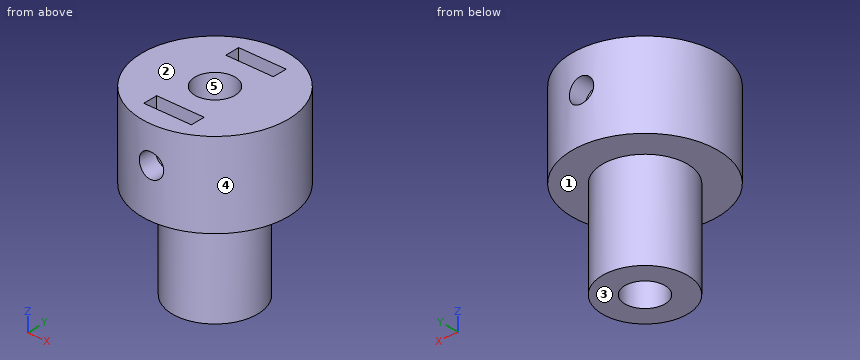
from build123d import *

# Parameters (mm, degrees)
SKETCH1_R           = 6
BOSS_EXTRUDE1_DEPTH = 15
SKETCH2_R           = 1.65
CUT_EXTRUDE1_DEPTH  = 18.23368794
SKETCH13_W          = 3.9
SKETCH13_H          = 1.2
CUT_EXTRUDE6_DEPTH  = 4.95
SKETCH4_R           = 1
CUT_EXTRUDE7_DEPTH  = 7.5
SKETCH19_R          = 6
SKETCH19_R_2        = 5.5
SKETCH19_R_3        = 3.5
CUT_EXTRUDE12_DEPTH = 8


with BuildPart() as part:
    # Sketch1 → Boss-Extrude1 (new body)
    with BuildSketch(Plane.XY):
        Circle(SKETCH1_R)
    extrude(amount=BOSS_EXTRUDE1_DEPTH)

    # Sketch2 → Cut-Extrude1 (cut, through all)
    with BuildSketch(Plane.XY.offset(15)):
        Circle(SKETCH2_R)
    extrude(amount=-CUT_EXTRUDE1_DEPTH, mode=Mode.SUBTRACT)

    # Sketch13 → Cut-Extrude6 (cut)
    with BuildSketch(Plane.XY.offset(15)):
        with Locations((0, 3.825)):
            Rectangle(SKETCH13_W, SKETCH13_H)
    cut_extrude6 = extrude(amount=-CUT_EXTRUDE6_DEPTH, mode=Mode.SUBTRACT)

    # Sketch4 → Cut-Extrude7 (cut, symmetric)
    with BuildSketch(Plane(origin=(0, 0, 0), x_dir=(1, 0, 0), z_dir=(0, 1, 0))):
        with Locations(Location((0, -12, 0), (0, 0, 270))):
            Circle(SKETCH4_R)
    extrude(amount=CUT_EXTRUDE7_DEPTH, both=True, mode=Mode.SUBTRACT)

    # Mirror1: Cut-Extrude6 across plane
    add(cut_extrude6.mirror(Plane.ZX), mode=Mode.SUBTRACT)

    # Sketch19 → Cut-Extrude12 (cut)
    # profile 1 of 2: a face of its own
    with BuildSketch(Plane(origin=(0, 0, 0), x_dir=(-1, 0, 0), z_dir=(0, 0, -1))):
        Circle(SKETCH19_R)
        Circle(SKETCH19_R_2, mode=Mode.SUBTRACT)
    # profile 2 of 2: a face of its own
    with BuildSketch(Plane(origin=(0, 0, 0), x_dir=(-1, 0, 0), z_dir=(0, 0, -1))):
        Circle(SKETCH19_R_2)
        Circle(SKETCH19_R_3, mode=Mode.SUBTRACT)
    extrude(amount=-CUT_EXTRUDE12_DEPTH, mode=Mode.SUBTRACT)


solid = part.part
Input: part model. Units: mm. Frame: model coordinates. Face numbers are marked on the shaded views. A direction names the side the tool comes from. Coordinates: 2 decimals unless noted, no trailing zeros. Write each loop counter-clockwise with the first axis right and the second up, starting at its lowest first coordinate (ties: lowest second). Pieces come first, ordered by that corner, then holes. Notation, with made-up numbers: M -22.75,10.5 L 26.25,10.5 A26 cw 26.25,37.5 Z; hole C 7,50 d9. An arc over 180 degrees is marked long. Answer as a JSON object with one key per item and string values. Group by question number.
(1) Ray query, line 1 along Y through (x, z) = (-1.5, 14.25) (3 decimals); line 2 along Y through (x, z) = (-0.5, 13.25) (3 decimals); line 3 along X through (y, z) = (-0.75, 9.5). Return the intervals inside material, ascending. Write a range as [from, to].
(2) Mould query, pull axis X, two halves, no side actions, for the marked faces 3, 4 and 5. Classes: pulls with the +X half, pulls with the -X half, needs draft (parallel to the pull), parting line crosses it, or undercut.
(3) Set-up query: the marked faces 1 and 2. Return all of +Z, -Z, +X, -X, +Y, -Y with unobstructed straight access to the full face (end or side cutting, diameter ignored); none if empty.
(4) Section A-A on y = 0. Output: boundary loops of the cut face in (x, z), plus the area to 3 significant figures.
(5) Section B-B on z = 12. Output: boundary loops of the cut face in (x, y) (3 decimals).
(6) Section C-C on x = 0. Give the number of separate pieces and of enclosed holes in the cut face, plus the area to 3 significant figures.
(7) Section D-D on z = 4.5. Output: boundary loops of the cut face in (x, y), plus the area to 3 significant figures.
(8) Contact query for flat-ended pins moving along their axis: P1, Ø1.2, axis at x = -0.5, z = 12, coming from the -Y side; P2, Ø2, axis at x = 2.5, z = 2.5, coming from the -Y side; P3, Ø0.6, axis at y = 3.5, z = 12.5, coming from the +X side. Output: stop coordinate, or through.
Result set:
{
 "1": {"line 1": "y = [-5.809, -4.425], [-3.225, -0.687], [0.687, 3.225], [4.425, 5.809]", "line 2": "y = [-5.979, -4.425], [-3.225, -1.572], [1.572, 3.225], [4.425, 5.979]", "line 3": "x = [-5.95, -1.47], [1.47, 5.95]"},
 "2": {"face 3": "needs draft", "face 4": "parting line crosses it", "face 5": "undercut"},
 "3": {"face 1": "-Z", "face 2": "+Z, +X, -X, +Y, -Y"},
 "4": {"outline": "M -6,8 L -3.5,8 L -3.5,0 L -1.65,0 L -1.65,15 L -6,15 Z; M 1.65,0 L 3.5,0 L 3.5,8 L 6,8 L 6,15 L 1.65,15 Z", "area": "90.5 mm2"},
 "5": {"outline": "M -1.95,-4.425 L -1.95,-3.225 L -1,-3.225 L -1,-1.312 A1.65 cw -1,1.312 L -1,3.225 L -1.95,3.225 L -1.95,4.425 L -1,4.425 L -1,5.916 A6 ccw -1,-5.916 L -1,-4.425 Z; M 1,-5.916 A6 ccw 1,5.916 L 1,4.425 L 1.95,4.425 L 1.95,3.225 L 1,3.225 L 1,1.312 A1.65 cw 1,-1.312 L 1,-3.225 L 1.95,-3.225 L 1.95,-4.425 L 1,-4.425 Z"},
 "6": {"separate pieces": "6", "enclosed holes": "0", "area": "66.0 mm2"},
 "7": {"outline": "C 0,0 d7; hole C 0,0 d3.3", "area": "29.9 mm2"},
 "8": {"P1": "stops at y = -5.93", "P2": "stops at y = -3.16", "P3": "stops at x = 5.08"}
}
